CAD build for the part. Positions are in the model's coordinates, mm. Face numbers are marked on the shaded views. A direction names the side the tool comes from. Give positions to 0.01 mm unless a question says otherwise; leave off trailing zeros. Write each loop counter-clockwise with the first axis right and the second up, starting at its lowest first coordinate (ties: lowest second). Pieces come first, ordered by that corner, then holes. Notation, with made-up numbers: (-28, 18) - (27, 18) arc R17 cw to (27, 36) - close; hole circle Ø3 at (46.25, 47). An arc over 180 degrees is marked (long way). Put each result on its own line as item: value. Start each with the question number.
1. Drop flat-ended pins along their axis: pin 1 (1.5 mm diameter, centred on x = -22, y = 0.5, fed in from +Z); pin 2 (1.8 mm diameter, centred on x = -37.5, y = -0.5, fed in from -Z); pin 3 (14 mm diameter, centred on x = -17.5, z = 168.5, fed in from +Y). Give the stop position or say it passes through.
2. Tool access for the marked faces 1 and 2: list every direction of +Z, -Z, +X, -X, +Y, -Y with a clear straight run to the whole face (end or side of a thin tool).
3. Wall check: line 1 (X direction, y = 12.25, z = 208.5); line 2 (Y direction, x = -49.5, z = 289); line 3 (Z direction, x = -6.5, y = -0.25). Give the ranges that are in metal, low to high.
4. Cut at B-B on x = -29. List the corners of the cut face in (y, z).
5. Cut at A-A on z = 190. List the corners of the cut face in (x, y), and give its area (3 significant figures).
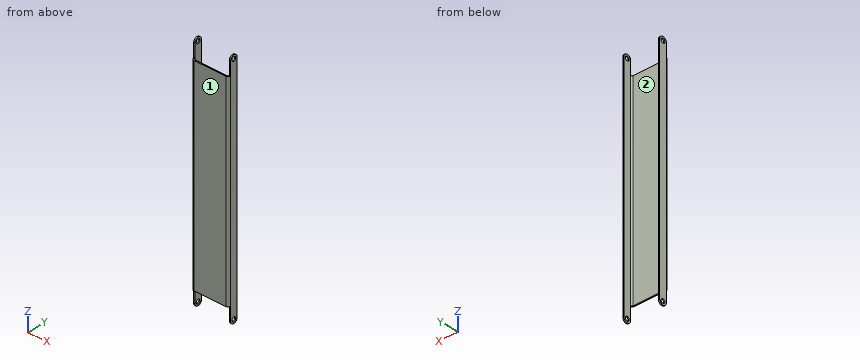
from build123d import *

# Parameters (mm, degrees)
F1_DEPTH = 304.8
F2_R     = 3.69316
F3_R     = 1.98374
F4_W     = 1.70942
F4_H     = 25.4
F6_DEPTH = 11.1125
F7_R     = 5.55624
F8_R     = 3.175
F9_DEPTH = 54.737


# Not quite as in the source:
# - a fillet or chamfer is up to 0.001 mm smaller than in the source, because OpenCascade refuses the exact size


with BuildPart() as f1:
    # F0 (on Top) → F1 (new body)
    with BuildSketch(Plane.XY):
        Polygon((0, 13.09624), (0, 0), (-51.31816, 0), (-51.31816, 13.09624), (-53.02758, 13.09624), (-53.02758, -1.70942), (1.70942, -1.70942), (1.70942, 13.09624), align=None)
    extrude(amount=F1_DEPTH)

    # F2
    f2_edges = [f1.edges().sort_by_distance(p)[0] for p in [
        (1.70942, -1.70942, 152.4),
        (-53.02758, -1.70942, 152.4),
    ]]
    fillet(f2_edges, radius=F2_R)

    # F3
    f3_edges = [f1.edges().sort_by_distance(p)[0] for p in [
        (0, 0, 152.4),
        (-51.31816, 0, 152.4),
    ]]
    fillet(f3_edges, radius=F3_R)

    # F4 (on face) → F6 (join, through all)
    with BuildSketch(Plane(origin=(0, 13.09624, 0), x_dir=(-1, 0, 0), z_dir=(0, 1, 0))):
        with Locations((52.17287, 317.5)):
            Rectangle(F4_W, F4_H)
        with Locations((-0.85471, 317.5)):
            Rectangle(F4_W, F4_H)
        with Locations((-0.85471, -12.7)):
            Rectangle(F4_W, F4_H)
        with Locations((52.17287, -12.7)):
            Rectangle(F4_W, F4_H)
    extrude(amount=-F6_DEPTH)

    # F7 (radius 5.55625 in the source; OpenCascade refuses exactly that, so slightly less here)
    f7_edges = [f1.edges().sort_by_distance(p)[0] for p in [
        (-52.17287, 13.09624, -25.4),
        (0.85471, 13.09624, -25.4),
        (0.85471, 13.09624, 330.2),
        (-52.17287, 13.09624, 330.2),
        (-52.17287, 1.98374, -25.4),
        (-52.17287, 1.98374, 330.2),
        (0.85471, 1.98374, 330.2),
        (0.85471, 1.98374, -25.4),
    ]]
    fillet(f7_edges, radius=F7_R)

    # F8 (on face) → F9 (cut, through all)
    with BuildSketch(Plane.YZ.offset(1.70942)):
        with Locations((7.53999, -19.84375)):
            Circle(F8_R)
        with Locations((7.53999, 324.64375)):
            Circle(F8_R)
    extrude(amount=-F9_DEPTH, mode=Mode.SUBTRACT)


solid = f1.part
Report:
1. pin 1: stops at z = 304.8
1. pin 2: stops at z = 0
1. pin 3: stops at y = 0
2. face 1: +Z, -Z, +X, -X, -Y
2. face 2: +Z, -Z, +Y
3. line 1: x = -53.03 to -51.32, 0 to 1.71
3. line 2: y = -1.71 to 0.01
3. line 3: z = 0 to 304.8
4. outline: (-1.71, 0) - (0, 0) - (0, 304.8) - (-1.71, 304.8) - close
5. outline: (-53.03, 1.98) arc R3.69 ccw to (-49.33, -1.71) - (-1.98, -1.71) arc R3.69 ccw to (1.71, 1.98) - (1.71, 13.1) - (0, 13.1) - (0, 1.98) arc R1.98 cw to (-1.98, 0) - (-49.33, 0) arc R1.98 cw to (-51.32, 1.98) - (-51.32, 13.1) - (-53.03, 13.1) - close
5. area: 134 mm²
